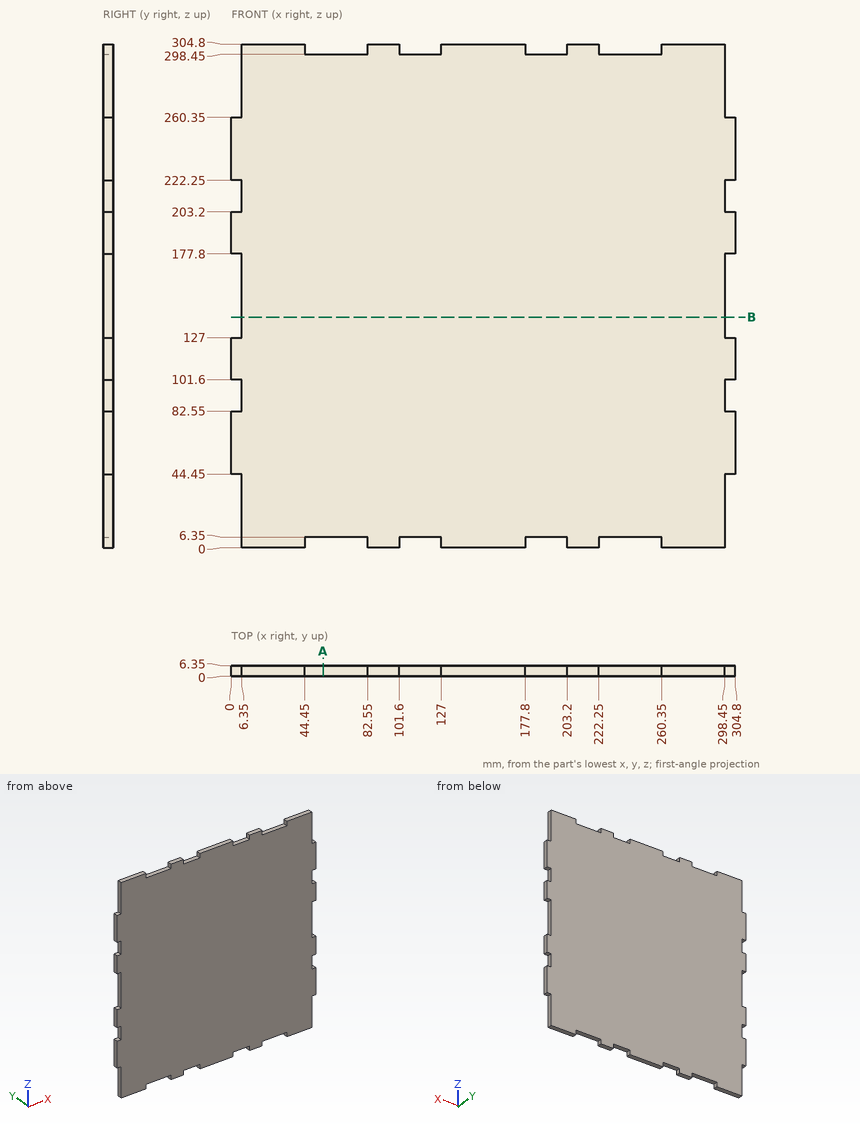
Geometry check sheet. Reference: drawing and pictorial views, mm from the part's lowest x, y, z. Round coordinates to 2 decimals unless told otherwise and drop trailing zeros. Write each loop counter-clockwise with the first axis right and the second up, starting at its lowest first coordinate (ties: lowest second). Pieces come first, ordered by that corner, then holes. Notation, with made-up numbers: (-13, 16) -> (12, 16) arc R26 ccw to (12, 37) -> close; hole circle Ø5 at (-18, -29.5). An arc over 180 degrees is marked (long way). One line per question, with ' | ' between items. Start each with the question number.
1. Sectioned sample at A-A, the plane x = 55.5. Record the cut outline in (y, z).
2. Depth check by flat-ended pin: pin 1 (4 mm diameter, centred on x = 54, z = 138.5, fed in from -Y); pin 2 (1.9 mm diameter, centred on y = 3.5, z = 14.5, fed in from +X); pin 3 (1.9 mm diameter, centred on y = 2, z = 21.5, fed in from -X); pin 4 (1.9 mm diameter, centred on x = 3.5, y = 3, fed in from +Z). Enter the tip coordinate at first touch or a pass-through.
3. Scan line: line 1 along Z through (x, y) = (57, 0.5). Record every from-to range of solid material in increasing order. Write a range as from..to.
4. Sectioned sample at B-B, the plane z = 139.5. Record the cut outline in (x, y), then the cut area to 3 significant figures.
Taken from the geometry:
1) outline: (0, 6.35) -> (6.35, 6.35) -> (6.35, 298.45) -> (0, 298.45) -> close
2) pin 1: stops at y = 0 | pin 2: stops at x = 298.45 | pin 3: stops at x = 6.35 | pin 4: stops at z = 260.35
3) line 1: z = 6.35..298.45
4) outline: (6.35, 0) -> (298.45, 0) -> (298.45, 6.35) -> (6.35, 6.35) -> close | area: 1,850 mm^2
